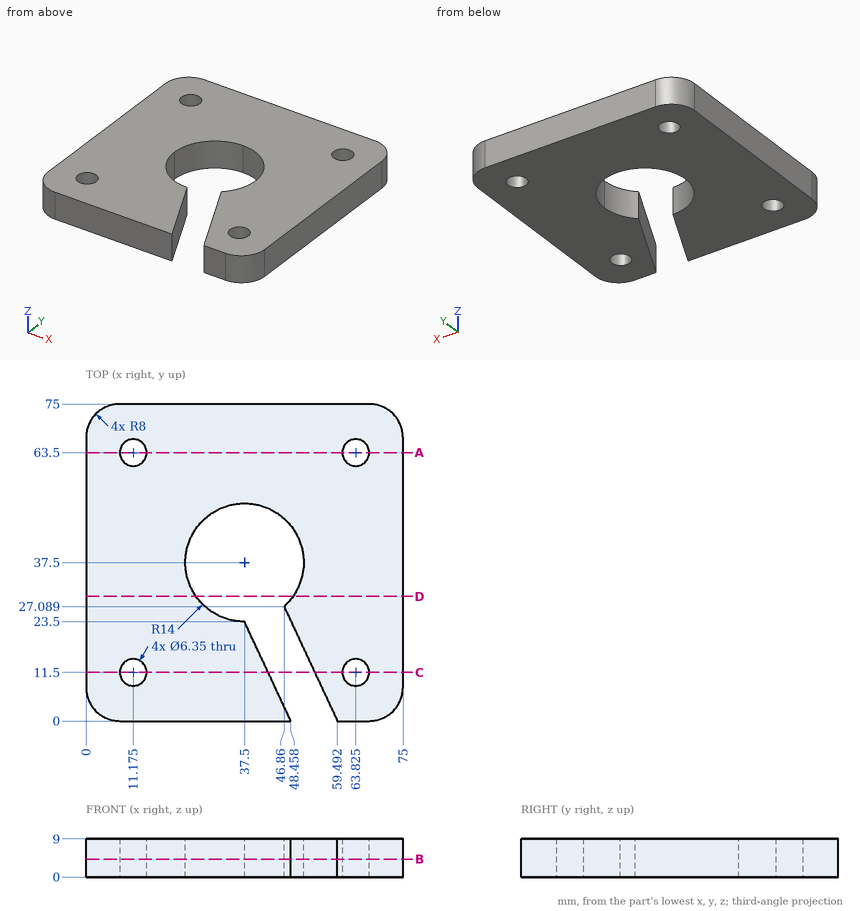
Source: three-view drawing plus pictorial views. Frame: mm from the lowest corner of the part. Round coordinates to 2 decimals unless told otherwise and drop trailing zeros. Loops run counter-clockwise (first coordinate to the right, second up) from the corner with the lowest first, then second, coordinate; pieces in that order, holes last. Notation, with made-up numbers: (4.25, 87) - (29.25, 87) arc R12 cw to (29.25, 103) - close; hole circle Ø4 at (8, 0.5). An arc over 180 degrees is marked (long way). Write each question's results on one line, items separated by ' | '. Start each with the question number.
1) Cut plane D-D on y = 29.5. Return loops of the section in (x, z).
2) Line query: probe 1 along X at (y, z) = (37, 5); probe 2 along Y at (x, z) = (35, 5.25) (1 decimal); probe 3 along Y at (x, z) = (47, 5) (1 decimal). Output: solid intervals per line, ascending. Write a range as [from, to].
3) Cut plane B-B on z = 4.25. Count the separate pieces of the cut face and the enclosed holes in it, then the cut area to 4 significant figures.
4) Cut plane C-C on y = 11.5. Return loops of the section in (x, z), then the cut area to 3 significant figures.
5) Cut plane A-A on y = 63.5. Return loops of the section in (x, z).
Verdict:
1) outline: (0, 0) - (26.01, 0) - (26.01, 9) - (0, 9) - close; (48.99, 0) - (75, 0) - (75, 9) - (48.99, 9) - close
2) probe 1: x = [0, 23.51], [51.49, 75] | probe 2: y = [0, 23.7], [51.3, 75] | probe 3: y = [0, 3.1], [26.8, 27.2], [47.8, 75]
3) separate pieces: 1 | enclosed holes: 4 | area: 4,555 mm2
4) outline: (0, 0) - (8, 0) - (8, 9) - (0, 9) - close; (14.35, 0) - (43.1, 0) - (43.1, 9) - (14.35, 9) - close; (54.13, 0) - (60.65, 0) - (60.65, 9) - (54.13, 9) - close; (67, 0) - (75, 0) - (75, 9) - (67, 9) - close | area: 461 mm2
5) outline: (0, 0) - (8, 0) - (8, 9) - (0, 9) - close; (14.35, 0) - (60.65, 0) - (60.65, 9) - (14.35, 9) - close; (67, 0) - (75, 0) - (75, 9) - (67, 9) - close
